Check sheet for the modelled part. Datum: model origin and axes. Units: mm. A direction names the side the tool comes from. Give positions to 0.01 mm unless a question says otherwise; leave off trailing zeros. Write each loop counter-clockwise with the first axis right and the second up, starting at its lowest first coordinate (ties: lowest second). Pieces come first, ordered by that corner, then holes. Notation, with made-up numbers: (0.25, 83) -> (50.25, 83) arc R20 cw to (50.25, 109) -> close; hole circle Ø10 at (-8.5, -13). An arc over 180 degrees is marked (long way). Return JSON: item names as keys, results as strings.
from build123d import *

# Parameters (mm, degrees)
F0_W     = 50
F0_H     = 70
F0_W_2   = 20
F0_H_2   = 40
F1_DEPTH = 10


with BuildPart() as f1:
    # F0 (on Front) → F1 (new body)
    with BuildSketch(Plane.XZ):
        with Locations((25, 35)):
            Rectangle(F0_W, F0_H)
        with Locations((30, 30)):
            Rectangle(F0_W_2, F0_H_2, mode=Mode.SUBTRACT)
    extrude(amount=-F1_DEPTH)


solid = f1.part
(1) Cross-section at B-B on z = 12. Enter the section's corners in (x, y).
Reply:
{"outline": "(0, 0) -> (20, 0) -> (20, 10) -> (0, 10) -> close; (40, 0) -> (50, 0) -> (50, 10) -> (40, 10) -> close"}
(2) Cross-section at C-C on y = 2. Enter the section's corners in (x, z).
Reply:
{"outline": "(0, 0) -> (50, 0) -> (50, 70) -> (0, 70) -> close; hole (20, 10) -> (40, 10) -> (40, 50) -> (20, 50) -> close"}
(3) Release check for a two-part mould opening along X. For faces 1 (the flat face through (50, 5, 35)), 2 (the flat face through (25, 5, 0)), 3 (the flat face through (30, 5, 10)) record: pulls with the +X half, pulls with the -X half, needs draft (parallel to the pull), parting line crosses it, or undercut.
Reply:
{"face 1": "pulls with the +X half", "face 2": "needs draft", "face 3": "undercut"}
(4) Cross-section at A-A on x = 22. Enter the section's corners in (y, z), then the cut area to 3 significant figures.
Reply:
{"outline": "(0, 0) -> (10, 0) -> (10, 10) -> (0, 10) -> close; (0, 50) -> (10, 50) -> (10, 70) -> (0, 70) -> close", "area": "300 mm^2"}
(5) Thickness scan on L1, parallel to Z at x = 36, y = 8.5; L2, parallel to X at y = 2.5, z = 11.5. Record the ranges inside material, lowest first.
Reply:
{"L1": "0 to 10, 50 to 70", "L2": "0 to 20, 40 to 50"}
(6) Set-up check for faces 4 (the flat face through (30, 5, 50)), 5 (the flat face through (25, 5, 70)): record each of +Z, -Z, +X, -X, +Y, -Y from which the full face is reachable in a straight line by a thin tool's end or side.
Reply:
{"face 4": "+Y, -Y", "face 5": "+Z, +X, -X, +Y, -Y"}
